Geometry check sheet. Reference: the model listing, model coordinates, mm. Coordinates: 2 decimals unless noted, no trailing zeros. Order: outer loops, then holes, each group sorted by start corner. A loop starts at its lowest first (then second) coordinate and runs counter-clockwise, first axis right, second up. Notation, with made-up numbers: M 16,18 L 20,18 A9 ccw 20,28 Z; hole C -12,30 d8. An arc over 180 degrees is marked long. One line per item, written item: value. Start each with the question number.
1) Sectioned sample at B-B, the plane z = -99. Enter the section's corners in (x, y).
2) Sectioned sample at C-C, the plane x = 126.5. Enter the section's corners in (y, z), then the cut area to 3 significant figures.
3) Sectioned sample at D-D, the plane x = 156. Enter the section's corners in (y, z).
4) Thickness scan on L1, parallel to X at y = 55, z = -68; L2, parallel to Z at x = 51.5, y = 76; L3, parallel to Z at x = 109, y = 3.5. Record the ranges inside material, lowest first. Write a range as from..to.
5) Go/stop test with flat-tipped pins: P1, Ø12, axis at x = 40.87, y = 9.65, coming from the -Z side; P2, Ø1, axis at x = 142.5, z = -113, coming from the +Y side; P3, Ø4, axis at y = 3, z = -27.5, coming from the +X side. Record where each tip stops, or that it passes through.
6) Sectioned sample at A-A, the plane y = 95.25. Enter the section's corners in (x, z).
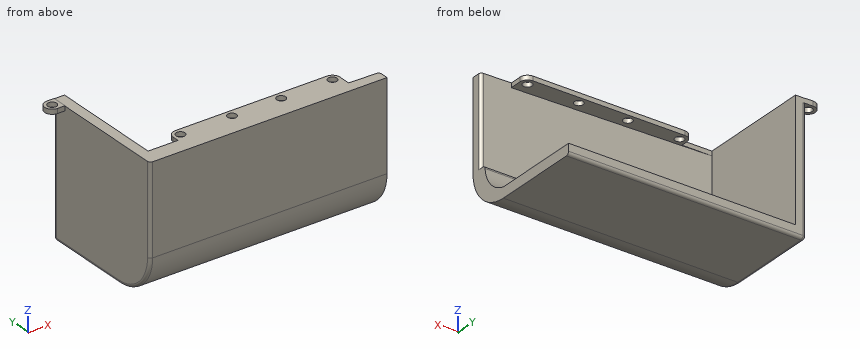
```python
from build123d import *

# Parameters (mm, degrees)
BOSS_EXTRUDE1_DEPTH      = 203.2
CUT_EXTRUDE1_DEPTH       = 194.31
CUT_EXTRUDE2_DEPTH       = 76.2
FILLET1_R                = 2.54
SKETCH8_R                = 3.793541353
BOSS_EXTRUDE2_DEPTH      = 3.81
BOSS_EXTRUDE3_DEPTH      = 0.254
BOSS_EXTRUDE3_DEPTH_BACK = 3.81
SKETCH9_R                = 3.815492591
FILLET2_R                = 2.54
FILLET4_R                = 2.54
FILLET5_R                = 2.54


with BuildPart() as part:
    # Sketch1 → Boss-Extrude1 (new body)
    with BuildSketch(Plane(origin=(0, 0, 0), x_dir=(0, 0, -1), z_dir=(1, 0, 0))):
        with BuildLine():
            Line((25.4, 0), (25.4, -10.16))
            Line((25.4, -10.16), (101.6, -10.16))
            ThreePointArc((101.6, -10.16), (126.744717139, 0.255282861), (137.16, 25.4))
            Line((137.16, 25.4), (137.16, 101.6))
            Line((137.16, 101.6), (127, 101.6))
            Line((127, 101.6), (25.4, 101.6))
            Line((25.4, 101.6), (25.4, 0))
        make_face()
    extrude(amount=BOSS_EXTRUDE1_DEPTH)

    # Sketch4 → Cut-Extrude1 (cut)
    with BuildSketch(Plane(origin=(203.2, 0, 0), x_dir=(0, 0, -1), z_dir=(1, 0, 0))):
        with BuildLine():
            Line((25.4, 3.81), (101.6, 3.81))
            ThreePointArc((101.6, 3.81), (118.756755229, 9.884008246), (128.27, 25.4))
            Line((128.27, 25.4), (128.27, 101.6))
            Line((128.27, 101.6), (25.4, 101.6))
            Line((25.4, 101.6), (25.4, 3.81))
        make_face()
    extrude(amount=-CUT_EXTRUDE1_DEPTH, mode=Mode.SUBTRACT)

    # Sketch5 → Cut-Extrude2 (cut)
    with BuildSketch(Plane.XY.offset(-25.4)):
        Polygon((203.2, 3.81), (8.89, 3.81), (203.2, -1.27), align=None)
    extrude(amount=-CUT_EXTRUDE2_DEPTH, mode=Mode.SUBTRACT)

    # Fillet1
    # the kernel refuses this fillet: 2.54 mm, written as the material it takes off along each edge
    with BuildSketch(Plane(origin=(209.278955694, 3.81, -101.6), x_dir=(0, -1, 0), z_dir=(-1, 0, 0))) as fillet1_piece_1_section:
        with BuildLine():
            CenterArc((2.431582278, -2.54), FILLET1_R, 90, 85.111724817)
            ThreePointArc((-0.099179119, -2.323558897), (-0.024806063, -1.162837311), (0, 0))
            Line((0, 0), (2.431582278, 0))
        make_face()
    fillet1_piece_1 = extrude(amount=200.388955694, mode=Mode.PRIVATE)
    fillet1_piece_1 = split(fillet1_piece_1, bisect_by=Plane(origin=(118.388821379, 0.947285716, -102.156943798), z_dir=(0.02613486081539205, 0.9996584261887458, 0)), keep=Keep.TOP, mode=Mode.PRIVATE)
    add(fillet1_piece_1, mode=Mode.SUBTRACT)

    # Sketch8 → Boss-Extrude2 (add)
    with BuildSketch(Plane.XY.offset(-25.4)):
        with BuildLine():
            Line((34.518861263, 3.823081405), (8.89, 3.81))
            Line((8.89, 3.81), (177.388856757, -0.595198869))
            Line((177.388856757, -0.595198869), (177.388856757, 9.645912611))
            ThreePointArc((177.388856757, 9.645912611), (175.528984934, 14.136040391), (171.038857154, 15.995912214))
            Line((171.038857154, 15.995912214), (40.868860866, 15.995912214))
            ThreePointArc((40.868860866, 15.995912214), (36.378733086, 14.136040391), (34.518861263, 9.645912611))
            Line((34.518861263, 9.645912611), (34.518861263, 3.823081405))
        make_face()
        with Locations((127.001989144, 9.496635092)):
            Circle(SKETCH8_R, mode=Mode.SUBTRACT)
        with Locations((171.038857154, 9.645912611)):
            Circle(SKETCH8_R, mode=Mode.SUBTRACT)
        with Locations((40.868860866, 9.645912611)):
            Circle(SKETCH8_R, mode=Mode.SUBTRACT)
        with Locations((85.055006395, 9.645912611)):
            Circle(SKETCH8_R, mode=Mode.SUBTRACT)
    extrude(amount=-BOSS_EXTRUDE2_DEPTH)

    # Sketch9 → Boss-Extrude3 (add, two sides: drawn at the far end of the back side and taken through both)
    with BuildSketch(Plane.XY.offset(-25.4).offset(-BOSS_EXTRUDE3_DEPTH_BACK)):
        with BuildLine():
            Line((0, 96.077095974), (0, 101.6))
            Line((0, 101.6), (-6.295904403, 101.6))
            ThreePointArc((-6.295904403, 101.6), (-12.645904403, 95.25), (-6.295904403, 88.9))
            Line((-6.295904403, 88.9), (0, 88.9))
            Line((0, 88.9), (0, 94.422904026))
            Line((0, 94.422904026), (0, 96.077095974))
        make_face()
        with Locations((-6.295904403, 95.25)):
            Circle(SKETCH9_R, mode=Mode.SUBTRACT)
    extrude(amount=BOSS_EXTRUDE3_DEPTH + BOSS_EXTRUDE3_DEPTH_BACK)

    # Fillet2
    fillet2_edges = [part.edges().sort_by_distance(p)[0] for p in [
        (101.6, 101.6, -137.16),
    ]]
    fillet(fillet2_edges, radius=FILLET2_R)

    # Fillet4
    fillet4_edges = [part.edges().sort_by_distance(p)[0] for p in [
        (203.2, -1.27, -63.5),
    ]]
    fillet(fillet4_edges, radius=FILLET4_R)

    # Fillet5
    fillet5_edges = [part.edges().sort_by_distance(p)[0] for p in [
        (0, 101.6, -81.915),
        (0, 100.856051224, -136.416051224),
        (0, 62.23, -137.16),
        (0, 0.255282861, -126.744717139),
        (0, -10.16, -63.5),
    ]]
    fillet(fillet5_edges, radius=FILLET5_R)


solid = part.part
```
Final values:
1. outline: M 0,-7.62 A2.54 ccw 2.54,-10.16 L 203.2,-10.16 L 203.2,-3.74 A2.54 ccw 200.73,-1.21 L 8.89,3.81 L 8.89,101.6 L 2.54,101.6 A2.54 ccw 0,99.06 Z
2. outline: M -10.16,-101.6 A35.56 ccw 25.4,-137.16 L 99.06,-137.16 A2.54 ccw 101.6,-134.62 L 101.6,-128.27 L 25.4,-128.27 A27.27 cw 3.91,-103.92 A2.54 ccw 1.38,-101.6 L 0.74,-101.6 L 0.74,-29.21 L 5.74,-29.21 L 5.74,-25.4 L -10.16,-25.4 Z; M 13.26,-29.21 L 16,-29.21 L 16,-25.4 L 13.26,-25.4 Z
2. area: 2,100 mm^2
3. outline: M -10.16,-101.6 A35.56 ccw 25.4,-137.16 L 99.06,-137.16 A2.54 ccw 101.6,-134.62 L 101.6,-128.27 L 25.4,-128.27 A27.27 cw 3.91,-103.92 A2.54 ccw 1.38,-101.6 L -0.04,-101.6 L -0.04,-29.21 L 16,-29.21 L 16,-25.4 L -10.16,-25.4 Z
4. L1: x = 0..8.89
4. L2: z = -137.16..-128.27
4. L3: z = -129.62..-102.74, -29.21..-25.4
5. P1: stops at z = -135.8
5. P2: stops at y = 6.54
5. P3: stops at x = 177.39
6. outline: M -12.65,-29.21 L -10.11,-29.21 L -10.11,-25.15 L -12.65,-25.15 Z; M -2.48,-29.21 L 0,-29.21 L 0,-134.62 A2.54 ccw 2.54,-137.16 L 203.2,-137.16 L 203.2,-128.27 L 8.89,-128.27 L 8.89,-25.4 L 0,-25.4 L 0,-25.15 L -2.48,-25.15 Z
